Work out the finished part from the listing and answer in its coordinate system (mm). A direction names the side the tool comes from. Give positions to 0.01 mm unless a question says otherwise; leave off trailing zeros. Order: outer loops, then holes, each group sorted by start corner. A loop starts at its lowest first (then second) coordinate and runs counter-clockwise, first axis right, second up. Notation, with made-up numbers: (49.5, -24) - (98.5, -24) arc R27 cw to (98.5, 1) - close; hole circle Ø11 at (75.5, 88.5). An arc over 180 degrees is marked (long way). Put each result on its own line as item: value.
Solid Edge part; units mm, degrees
sketch "Sketch1" plane through (0, 0, 0) normal (0, 0, 1) x (1, 0, 0)
  circle A0 centre (-41.5111, 10.3403) radius 15
  line L0 (-91.5111, 135.3403) -> (-91.5111, -114.6597)
  line L1 (-91.5111, -114.6597) -> (8.4889, -114.6597)
  line L2 (8.4889, -114.6597) -> (8.4889, 135.3403)
  line L3 (8.4889, 135.3403) -> (-91.5111, 135.3403)
  dimension "D1" = 8.4889
  dimension "D2" = 91.5111
extrude "Protrusion1" add sketch "Sketch1" along normal blind 20
sketch "Sketch2" plane through (-51.5111, 20.3403, 0) normal (0, 0, -1) x (0, -1, 0)
  circle A0 centre (-100, -30) radius 4
  circle A1 centre (-70, 10) radius 4
  circle A2 centre (-70, -30) radius 4
  circle A3 centre (-100, 10) radius 4
  dimension "D1" = 100
extrude "Cutout1" cut sketch "Sketch2" against normal through all
mirror "Mirror1" about plane through (-51.5111, 10.3403, 5) normal (0, 1, 0) of "Cutout1"
sketch "Sketch3" plane through (-46.5111, 10.3403, 20) normal (0, 0, 1) x (1, 0, 0)
  circle A0 centre (5, 30) radius 6.1
extrude "Cutout3" cut sketch "Sketch3" against normal through all
sketch "Sketch4" plane through (-41.5111, 10.3403, 20) normal (0, 0, 1) x (1, 0, 0)
  circle A0 centre (0, 30) radius 10
extrude "Cutout4" cut sketch "Sketch4" against normal blind 8
pattern_circular "Pattern1" count 8 over 360 about axis through (-41.5111, 10.3403, 20) along (0, 0, -1) of "Cutout3", "Cutout4"
sketch "Sketch5" plane through (-41.5111, 10.3403, 0) normal (0, 0, -1) x (0, 1, 0)
  circle A0 centre (0, 0) radius 40
extrude "ExtrudedCutout_14" cut sketch "Sketch5" against normal blind 3
properties material "Aluminum, 6061-T6"
(1) Determine the mould class of faces 4 (the face through (-20.731, 41.544, 16.056)), 5 (the face through (8.489, 9, 10)) for opening direction Y: pulls with the +Y half, pulls with the -Y half, needs draft (parallel to the pull), parting line crosses it, or undercut.
Geometry check:
face 4: undercut
face 5: needs draft
(2) Section A-A, the plane x = -8 is taken. Write down the section's boundary in (y, z), then the cut area to 3 significant figures.
Geometry check:
outline: (-114.66, 0) - (-11.5, 0) - (-11.5, 3) - (5.35, 3) - (5.35, 12) - (0.98, 12) - (0.98, 20) - (-114.66, 20) - close; (15.33, 3) - (32.18, 3) - (32.18, 0) - (135.34, 0) - (135.34, 20) - (19.7, 20) - (19.7, 12) - (15.33, 12) - close
area: 4,630 mm²
(3) Section B-B, the plane z = 9 is taken. Count the separate pieces of the cut face and the enclosed holes in it, then the cut area to 3 significant figures.
Geometry check:
separate pieces: 1
enclosed holes: 17
area: 23,000 mm²
(4) Straight lines are drawn through the part: line 1 (X direction, y = -100, z = 10.5); line 2 (X direction, y = 2, z = 12.5); line 3 (X direction, y = -99, z = 5.75). For each, find the intervals that lie inside material, in ascending order.
Geometry check:
line 1: x = -91.51 to -65.5, -57.53 to -25.5, -17.53 to 8.49
line 2: x = -91.51 to -77.03, -65.99 to -53.98, -29.04 to -17.03, -5.99 to 8.49
line 3: x = -91.51 to -65.46, -57.57 to -25.46, -17.57 to 8.49
(5) A tool of negligible diameter and unlimited length cuts with its end or side. For faces 1 (the face through (-59, 11, 3)), 2 (the face through (-58.1, 40.42, 16.06)), 3 (the face through (-19.979, 116.645, 9.86)), from which of +Z, -Z, +X, -X, +Y, -Y can it reach the whole face along a straight path? Write none if from no direction.
Geometry check:
face 1: -Z
face 2: +Z
face 3: +Z, -Z
(6) Given pin 1 (14 mm diameter, centred on x = -41.51, y = -19.66, fed in from -Z); pin 2 (6 mm diameter, centred on x = -65.5, y = 36.5, fed in from +Z); pin 3 (7.5 mm diameter, centred on x = -71.51, y = 10.34, fed in from +Z), each flat-ended and moving along its own axis, determine where each tip first touches the part or whether it passes through.
Geometry check:
pin 1: stops at z = 3
pin 2: stops at z = 12
pin 3: passes through
(7) Section C-C, the plane x = -75 is taken. Write down the section's boundary in (y, z).
Geometry check:
outline: (-114.66, 0) - (-11.53, 0) - (-11.53, 3) - (5.34, 3) - (5.34, 12) - (0.97, 12) - (0.97, 20) - (-114.66, 20) - close; (15.34, 3) - (32.21, 3) - (32.21, 0) - (135.34, 0) - (135.34, 20) - (19.71, 20) - (19.71, 12) - (15.34, 12) - close
